Model file for the job. Use its own axes, mm. Face numbers are marked on the shaded views. Round coordinates to 2 decimals unless told otherwise and drop trailing zeros. Loops run counter-clockwise (first coordinate to the right, second up) from the corner with the lowest first, then second, coordinate; pieces in that order, holes last.
Autodesk Inventor part; units mm, degrees
ref_plane "Work Plane1" through (0, 0, 20) normal (0, 0, 1) x (1, 0, 0)
ref_plane "YZ Plane" through (0, 0, 0) normal (1, 0, 0) x (0, 1, 0)
ref_plane "XZ Plane" through (0, 0, 0) normal (0, 1, 0) x (-1, 0, 0)
sketch "Sketch1" plane through (0, 0, 0) normal (0, 0, 1) x (1, 0, 0)
  line L0 (-80, 463) -> (80, 463)
  line L1 (80, 463) -> (80, -463)
  line L2 (80, -463) -> (-80, -463)
  line L3 (-80, -463) -> (-80, 463)
  line L4 (0, 144.4625) -> (0, -193.675)
  line L5 (-174.625, 0) -> (185.7375, 0)
  point P0 (0, 0)
  dimension "d0" = 160
  dimension "d1" = 926
extrude "Extrusion1" add sketch "Sketch1" along normal blind 20
ref_plane "Work Plane1" through (0, 0, 20) normal (0, 0, 1) x (1, 0, 0)
sketch "Sketch2" plane through (0, 0, 20) normal (0, 0, 1) x (1, 0, 0)
  line L0 (-78.9983, 421.7822) -> (81.0017, 421.7822)
  line L1 (81.0017, 421.7822) -> (81.0017, 221.7822)
  line L2 (81.0017, 221.7822) -> (-78.9983, 221.7822)
  line L3 (-78.9983, 221.7822) -> (-78.9983, 421.7822)
  point P0 (0, 0)
  dimension "d5" = 200
  dimension "d6" = 160
extrude "Extrusion2" add sketch "Sketch2" along normal blind 20
sketch "Sketch3" plane through (0, 0, 20) normal (0, 0, 1) x (1, 0, 0)
  line L0 (-81.0461, -229.4574) -> (78.9539, -229.4574)
  line L1 (78.9539, -229.4574) -> (78.9539, -462.4574)
  line L2 (78.9539, -462.4574) -> (-81.0461, -462.4574)
  line L3 (-81.0461, -462.4574) -> (-81.0461, -229.4574)
  point P0 (0, 0)
  dimension "d9" = 233
  dimension "d10" = 160
extrude "Extrusion3" add sketch "Sketch3" along normal blind 40
properties part number "USW16T"
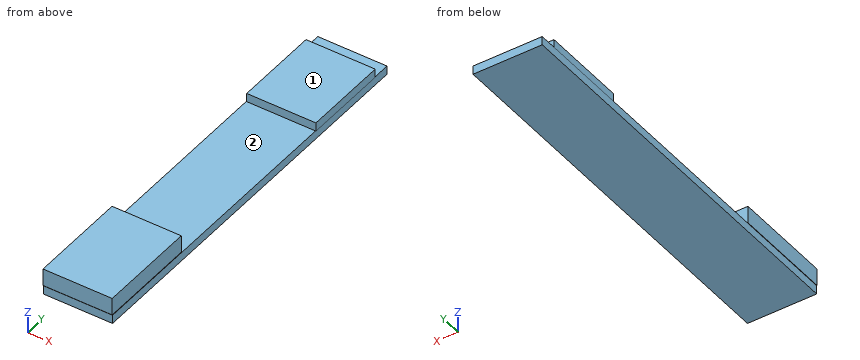
Q1. Flat gauge pins, fed straight in: P1, Ø2, axis at y = -198, z = 13, coming from the +X side; P2, Ø6, axis at y = 318, z = 29, coming from the -X side; P3, Ø0.8, axis at x = -80.5, y = -325.5, coming from the -Z side. Where does each tip first touch, or does it go through?
Q2. Slice it at A-A on z = 31. Give the cut face in (x, y), plus the area to 3 significant figures.
Q3. Slice it at B-B on y = 293. Give the cut face in (x, z).
Q4. Slice it at D-D on y = -199. Give the cut face in (x, z), plus the area to 3 significant figures.
Q5. Probe line 1 (Y direction, x = -34, z = 34); line 2 (Z direction, x = -49, y = 65.5); line 3 (X direction, y = 237, z = 30). List the from-to ranges inside material, lowest first.
Q6. Slice it at C-C on x = -39. Give the cut face in (y, z), plus the area to 3 significant figures.
Q7. Pull direction Y, two halves, no side cores. Call the marked faces 1 and 2: pulls with the +Y half, pulls with the -Y half, needs draft (parallel to the pull), parting line crosses it, or undercut.
Reply:
1. P1: stops at x = 80
1. P2: stops at x = -79
1. P3: stops at z = 20
2. outline: (-81.05, -462.46) - (78.95, -462.46) - (78.95, -229.46) - (-81.05, -229.46) - close; (-79, 221.78) - (81, 221.78) - (81, 421.78) - (-79, 421.78) - close
2. area: 69,300 mm2
3. outline: (-80, 0) - (80, 0) - (80, 20) - (81, 20) - (81, 40) - (-79, 40) - (-79, 20) - (-80, 20) - close
4. outline: (-80, 0) - (80, 0) - (80, 20) - (-80, 20) - close
4. area: 3,200 mm2
5. line 1: y = -462.46 to -229.46, 221.78 to 421.78
5. line 2: z = 0 to 20
5. line 3: x = -79 to 81
6. outline: (-463, 0) - (463, 0) - (463, 20) - (421.78, 20) - (421.78, 40) - (221.78, 40) - (221.78, 20) - (-229.46, 20) - (-229.46, 60) - (-462.46, 60) - (-462.46, 20) - (-463, 20) - close
6. area: 31,800 mm2
7. face 1: needs draft
7. face 2: undercut
